Part model, mm, in its own coordinate system. A direction names the side the tool comes from. Give positions to 0.01 mm unless a question says otherwise; leave off trailing zeros. Write each loop counter-clockwise with the first axis right and the second up, starting at its lowest first coordinate (ties: lowest second). Pieces come first, ordered by that corner, then holes. Notation, with made-up numbers: M 53.25,56.5 L 65.25,56.5 A17 ccw 65.25,73.5 Z; hole C 43,69.25 d7. An arc over 180 degrees is marked long. Answer as CSV lines item,"result". Start each with the question number.
1) Slice it at B-B, the plane x = 36. Give the cut face in (y, z), plus the area to 3 significant figures.
2) Slice it at A-A, the plane y = 57.5. Give the cut face in (x, z), plus the area to 3 significant figures.
3) Mould opens along Y. For faces 1 (the flat face through (0, 57, 2)), 2 (the cylindrical face through (1.711, 113.196, 2.028)), 3 (the flat face through (36, 63, 2)) say: pulls with the +Y half, pulls with the -Y half, needs draft (parallel to the pull), parting line crosses it, or undercut.
4) Slice it at D-D, the plane y = 32.5. Give the cut face in (x, z).
5) Slice it at C-C, the plane z = 2.25. Give the cut face in (x, y), plus the area to 3 significant figures.
6) Tool access for faces 4 (the flat face through (57, 58, 0)), 5 (the cylindrical face through (53, 38, 2)): list every direction of +Z, -Z, +X, -X, +Y, -Y with a clear straight run to the whole face (end or side of a thin tool).
7) Pin check, flat tip, straight feed: pin 1 Ø2.5 at (x, y) = (81, 27) entering from -Z. Stop position of the tip, or through.
8) Wall check: line 1 along Y through (x, z) = (81, 2.05); line 2 along Y through (x, z) = (24.5, 2); line 3 along X through (y, z) = (55, 0.4). Give the ranges that are in metal, low to high. Write a range as from..to.
```python
from build123d import *

# Parameters (mm, degrees)
F0_W     = 116
F0_H     = 115
F0_R     = 2
F0_W_2   = 10
F0_H_2   = 24
F1_DEPTH = 4
F2_R     = 6
F4_R     = 2
F4_R_2   = 17
F5_DEPTH = 25
F6_W     = 27.550638
F6_H     = 3.205147
F6_W_2   = 29.028984
F6_H_2   = 3.037915
F6_W_3   = 33.224199
F6_H_3   = 3
F7_DEPTH = 4


with BuildPart() as f1:
    # F0 (on Top) → F1 (new body)
    with BuildSketch(Plane.XY):
        with Locations((58, 57.5)):
            Rectangle(F0_W, F0_H)
        with Locations((81, 27)):
            Circle(F0_R, mode=Mode.SUBTRACT)
        with Locations((81, 57)):
            Rectangle(F0_W_2, F0_H_2, mode=Mode.SUBTRACT)
        with Locations((81, 88)):
            Circle(F0_R, mode=Mode.SUBTRACT)
    extrude(amount=F1_DEPTH)

    # F2
    f2_edges = [f1.edges().sort_by_distance(p)[0] for p in [
        (0, 115, 2),
        (116, 115, 2),
        (116, 0, 2),
        (0, 0, 2),
    ]]
    fillet(f2_edges, radius=F2_R)

    # F4 (on Top) → F5 (cut)
    with BuildSketch(Plane.XY):
        with Locations((36, 57.5)):
            Circle(F4_R)
        with Locations((36, 77)):
            Circle(F4_R_2)
        with Locations((36, 38)):
            Circle(F4_R_2)
    extrude(amount=F5_DEPTH, mode=Mode.SUBTRACT)

    # F6 (on face) → F7 (join)
    with BuildSketch(Plane.XY.offset(4)):
        Polygon((32.74464, 94.836249), (25.32669, 91), (46.063566, 91), (43.255925, 94.420469), align=None)
        with Locations((37.412647, 61.397426)):
            Rectangle(F6_W, F6_H)
        with Locations((37.197317, 53.518957)):
            Rectangle(F6_W_2, F6_H_2)
        with Locations((36.739217, 22.5)):
            Rectangle(F6_W_3, F6_H_3)
    extrude(amount=-F7_DEPTH)


solid = f1.part
```
Found:
1,outline,"M 0,0 L 24,0 L 24,4 L 0,4 Z; M 52,0 L 55.5,0 L 55.5,4 L 52,4 Z; M 59.5,0 L 63,0 L 63,4 L 59.5,4 Z; M 91,0 L 115,0 L 115,4 L 91,4 Z"
1,area,"220 mm²"
2,outline,"M 0,0 L 34,0 L 34,4 L 0,4 Z; M 38,0 L 76,0 L 76,4 L 38,4 Z; M 86,0 L 116,0 L 116,4 L 86,4 Z"
2,area,"408 mm²"
3,face 1,"needs draft"
3,face 2,"pulls with the +Y half"
3,face 3,"undercut"
4,outline,"M 0,0 L 19.91,0 L 19.91,4 L 0,4 Z; M 52.09,0 L 116,0 L 116,4 L 52.09,4 Z"
5,outline,"M 0,6 A6 ccw 6,0 L 110,0 A6 ccw 116,6 L 116,109 A6 ccw 110,115 L 6,115 A6 ccw 0,109 Z; hole M 26.36,24 L 45.64,24 A17 ccw 45.64,52 L 26.36,52 A17 ccw Z; hole M 26.36,63 L 45.64,63 A17 ccw 45.64,91 L 26.36,91 A17 ccw Z; hole C 36,57.5 d4; hole M 76,45 L 86,45 L 86,69 L 76,69 Z; hole C 81,27 d4; hole C 81,88 d4"
5,area,"11,400 mm²"
6,face 4,"-Z, +X, -X, +Y, -Y"
6,face 5,"+Z, -Z"
7,pin 1,"through"
8,line 1,"0..25, 29..45, 69..86, 90..115"
8,line 2,"0..25.48, 50.52..64.48, 89.52..115"
8,line 3,"0..76, 86..116"
